Part model, mm, in its own coordinate system. A direction names the side the tool comes from. Round coordinates to 2 decimals unless told otherwise and drop trailing zeros. Order: outer loops, then holes, each group sorted by start corner. A loop starts at its lowest first (then second) coordinate and runs counter-clockwise, first axis right, second up. Notation, with made-up numbers: M 22.5,5 L 66.5,5 A26 ccw 66.5,40 Z; hole C 34,88.25 d4. An arc over 180 degrees is marked long. Write each question's results on one line, items separated by ' | '. Start each with the question number.
1. Drop flat-ended pins along their axis: pin 1 Ø3 at (x, y) = (2, 31.5) entering from +Z; pin 2 Ø1 at (x, z) = (6, 39) entering from +Y; pin 3 Ø4 at (x, y) = (2, -27) entering from -Z. Give the stop position or say it passes through.
2. Two-plate mould, pull along Z, no slides. Class faces 4 (the face through (6.604, -28.842, 28.993)), 5 (the face through (6, 3.1, -39)), 6 (the face through (5, -10, -38)): +Z half, -Z half, draft (parallel to the pull), parting line (faces both ways), or undercut.
3. Which spindle directions (+Z, -Z, +X, -X, +Y, -Y) get a long thin tool onto all of the face, cutting with end or side? Do faces 1 (the face through (6, -37.1, -13.2)), 2 (the face through (6, 33.9, 0.1)), 3 (the face through (5, -33, -20)). Say none if no direction does.
4. Probe L1, parallel to Y at x = 2.6, z = 0; L2, parallel to Z at x = 2, y = 18; L3, parallel to Y at x = 1.75, z = -36. List the from-to ranges inside material, lowest first. Write a range as [from, to].
5. Band-saw the part on A-A, the plane z = 0. List the corners of the cut face in (x, y), then the cut area to 3 significant figures.
```python
from build123d import *

# Parameters (mm, degrees)
SKETCH_1_R                = 41.5
SKETCH_1_R_2              = 33.1
EXTRUDE_1_DEPTH           = 7
SKETCH_2_R                = 1.55
CUT_EXTRUDE_1_DEPTH       = 8
PATTERN_CIRCULAR_1_COUNT  = 12
SKETCH_3_R                = 33.1
SKETCH_3_R_2              = 29.5
EXTRUDE_2_DEPTH           = 2.5
CHAMFER_1_SIZE            = 1
SKETCH_4_R                = 1.55
CUT_EXTRUDE_8_DEPTH       = 2
PATTERN_CIRCULAR_7_COUNT  = 12
SKETCH_7_R                = 1.6
CUT_EXTRUDE_10_DEPTH      = 10
PATTERN_CIRCULAR_9_COUNT  = 4
PATTERN_CIRCULAR_9_ANGLE  = 90
SKETCH_6_R                = 3
CUT_EXTRUDE_9_DEPTH       = 3.5
PATTERN_CIRCULAR_8_COUNT  = 4
PATTERN_CIRCULAR_8_ANGLE  = 90
SKETCH_8_R                = 1.6
CUT_EXTRUDE_11_DEPTH      = 2
PATTERN_CIRCULAR_10_COUNT = 4
PATTERN_CIRCULAR_10_ANGLE = 90


with BuildPart() as part:
    # 草图1 → 凸台-拉伸1 (new body)
    with BuildSketch(Plane(origin=(0, 0, 0), x_dir=(0, 0, -1), z_dir=(1, 0, 0))):
        Circle(SKETCH_1_R)
        Circle(SKETCH_1_R_2, mode=Mode.SUBTRACT)
    extrude(amount=EXTRUDE_1_DEPTH)

    # 草图2 → 切除-拉伸1 (cut)
    with BuildSketch(Plane.ZY):
        with Locations((0, 37)):
            Circle(SKETCH_2_R)
    cut_extrude_1 = extrude(amount=-CUT_EXTRUDE_1_DEPTH, mode=Mode.SUBTRACT)

    # 阵列(圆周)1: 切除-拉伸1 ×12 about axis
    pattern_circular_1_axis = Axis((0, 0, 0), (1, 0, 0))
    for i in range(1, PATTERN_CIRCULAR_1_COUNT):
        add(cut_extrude_1.rotate(pattern_circular_1_axis, i * 360 / PATTERN_CIRCULAR_1_COUNT), mode=Mode.SUBTRACT)

    # 草图3 → 凸台-拉伸2 (add)
    with BuildSketch(Plane(origin=(7, 0, 0), x_dir=(0, 0, -1), z_dir=(1, 0, 0))):
        Circle(SKETCH_3_R)
        Circle(SKETCH_3_R_2, mode=Mode.SUBTRACT)
    extrude(amount=-EXTRUDE_2_DEPTH)

    # 倒角1
    chamfer_1_edges = [part.edges().sort_by_distance(p)[0] for p in [
        (7, 0, 41.5),
    ]]
    chamfer(chamfer_1_edges, length=CHAMFER_1_SIZE)

    # 草图4 → 切除-拉伸8 (cut)
    with BuildSketch(Plane(origin=(7, 0, 0), x_dir=(0, 0, -1), z_dir=(1, 0, 0))):
        with BuildLine():
            Line((40.381183737, 3.1), (37, 3.1))
            ThreePointArc((37, 3.1), (33.9, 0), (37, -3.1))
            Line((37, -3.1), (40.381183737, -3.1))
            ThreePointArc((40.381183737, -3.1), (40.470285033, -1.551138074), (40.5, 0))
            ThreePointArc((40.5, 0), (40.470285033, 1.551138074), (40.381183737, 3.1))
        make_face()
        with Locations((37, 0)):
            Circle(SKETCH_4_R, mode=Mode.SUBTRACT)
        with BuildLine():
            Line((41.5, 3.1), (40.381183737, 3.1))
            ThreePointArc((40.381183737, 3.1), (40.470285033, 1.551138074), (40.5, 0))
            ThreePointArc((40.5, 0), (40.470285033, -1.551138074), (40.381183737, -3.1))
            Line((40.381183737, -3.1), (41.5, -3.1))
            ThreePointArc((41.5, -3.1), (44.6, 0), (41.5, 3.1))
        make_face()
    cut_extrude_8 = extrude(amount=-CUT_EXTRUDE_8_DEPTH, mode=Mode.SUBTRACT)

    # 阵列(圆周)7: 切除-拉伸8 ×12 about axis
    pattern_circular_7_axis = Axis((0, 0, 0), (1, 0, 0))
    for i in range(1, PATTERN_CIRCULAR_7_COUNT):
        add(cut_extrude_8.rotate(pattern_circular_7_axis, i * 360 / PATTERN_CIRCULAR_7_COUNT), mode=Mode.SUBTRACT)

    # 草图7 → 切除-拉伸10 (cut)
    with BuildSketch(Plane.ZY):
        with Locations((-9.576304669, -35.739255573)):
            Circle(SKETCH_7_R)
    cut_extrude_10 = extrude(amount=-CUT_EXTRUDE_10_DEPTH, mode=Mode.SUBTRACT)

    # 阵列(圆周)9: 切除-拉伸10 ×4 about axis
    pattern_circular_9_axis = Axis((0, 0, 0), (1, 0, 0))
    for i in range(1, PATTERN_CIRCULAR_9_COUNT):
        add(cut_extrude_10.rotate(pattern_circular_9_axis, i * PATTERN_CIRCULAR_9_ANGLE / (PATTERN_CIRCULAR_9_COUNT - 1)), mode=Mode.SUBTRACT)

    # 草图6 → 切除-拉伸9 (cut)
    with BuildSketch(Plane.ZY):
        with Locations((-9.576304669, -35.739255573)):
            Circle(SKETCH_6_R)
    cut_extrude_9 = extrude(amount=-CUT_EXTRUDE_9_DEPTH, mode=Mode.SUBTRACT)

    # 阵列(圆周)8: 切除-拉伸9 ×4 about axis
    pattern_circular_8_axis = Axis((0, 0, 0), (1, 0, 0))
    for i in range(1, PATTERN_CIRCULAR_8_COUNT):
        add(cut_extrude_9.rotate(pattern_circular_8_axis, i * PATTERN_CIRCULAR_8_ANGLE / (PATTERN_CIRCULAR_8_COUNT - 1)), mode=Mode.SUBTRACT)

    # 草图8 → 切除-拉伸11 (cut)
    with BuildSketch(Plane(origin=(7, 0, 0), x_dir=(0, 0, -1), z_dir=(1, 0, 0))):
        with BuildLine():
            ThreePointArc((38.889255573, 9.576304669), (37.656854074, 12.075367691), (34.923975581, 12.618971022))
            ThreePointArc((34.923975581, 12.618971022), (32.69658922, 8.761024677), (36.554535565, 6.533638316))
            ThreePointArc((36.554535565, 6.533638316), (38.238318595, 7.658706167), (38.889255573, 9.576304669))
        make_face()
        with Locations((35.739255573, 9.576304669)):
            Circle(SKETCH_8_R, mode=Mode.SUBTRACT)
        with BuildLine():
            Line((40.719530538, 14.171885292), (34.923975581, 12.618971022))
            ThreePointArc((34.923975581, 12.618971022), (37.656854074, 12.075367691), (38.889255573, 9.576304669))
            ThreePointArc((38.889255573, 9.576304669), (38.238318595, 7.658706167), (36.554535565, 6.533638316))
            Line((36.554535565, 6.533638316), (42.350090523, 8.086552587))
            Line((42.350090523, 8.086552587), (40.719530538, 14.171885292))
        make_face()
    cut_extrude_11 = extrude(amount=-CUT_EXTRUDE_11_DEPTH, mode=Mode.SUBTRACT)

    # 阵列(圆周)10: 切除-拉伸11 ×4 about axis
    pattern_circular_10_axis = Axis((0, 0, 0), (-1, 0, 0))
    for i in range(1, PATTERN_CIRCULAR_10_COUNT):
        add(cut_extrude_11.rotate(pattern_circular_10_axis, i * PATTERN_CIRCULAR_10_ANGLE / (PATTERN_CIRCULAR_10_COUNT - 1)), mode=Mode.SUBTRACT)


solid = part.part
```
Solution:
1) pin 1: z = 28.67 | pin 2: y = 15.49 | pin 3: z = -33.12
2) face 4: +Z half | face 5: draft | face 6: undercut
3) face 1: +X, -Y | face 2: +X, +Y | face 3: +X
4) L1: [-41.5, -38.55], [-35.45, -33.1], [33.1, 35.45], [38.55, 41.5] | L2: [-37.39, -33.51], [-30.58, -27.78], [27.78, 30.58], [33.51, 37.39] | L3: [-20.65, -12.56], [-6.59, -1.18], [1.18, 6.59], [12.56, 20.65]
5) outline: M 0,-41.5 L 5,-41.5 L 5,-38.55 L 0,-38.55 Z; M 0,-35.45 L 5,-35.45 L 5,-33.9 L 7,-33.9 L 7,-29.5 L 4.5,-29.5 L 4.5,-33.1 L 0,-33.1 Z; M 0,33.1 L 4.5,33.1 L 4.5,29.5 L 7,29.5 L 7,33.9 L 5,33.9 L 5,35.45 L 0,35.45 Z; M 0,38.55 L 5,38.55 L 5,41.5 L 0,41.5 Z | area: 74.2 mm^2
